Read the model definition and answer for the solid it produces. Units are mm, in the model's axes. Give positions to 0.01 mm unless a question says otherwise; leave off trailing zeros. Loops run counter-clockwise (first coordinate to the right, second up) from the corner with the lowest first, then second, coordinate; pieces in that order, holes last. Notation, with made-up numbers: (-9, 34) -> (48, 34) arc R38 ccw to (48, 73) -> close; hole circle Ø11 at (15.5, 24). An arc over 180 degrees is marked (long way). Return JSON: item names as keys, results as strings. Group by question number.
from build123d import *

# Parameters (mm, degrees)
SKETCH1_W           = 185
SKETCH1_H           = 100
SKETCH1_W_2         = 122
SKETCH1_H_2         = 30
BOSS_EXTRUDE1_DEPTH = 5
CUT_EXTRUDE2_REACH  = 7
SKETCH2_R           = 1.6
CUT_EXTRUDE3_REACH  = 7
SKETCH3_R           = 1.6
CUT_EXTRUDE4_REACH  = 7
SKETCH4_R           = 1.6
CUT_EXTRUDE5_REACH  = 7
SKETCH5_R           = 1.6


with BuildPart() as part:
    # Sketch1 → Boss-Extrude1 (new body)
    with BuildSketch(Plane(origin=(0, 0, 0), x_dir=(1, 0, 0), z_dir=(0, 1, 0))):
        with Locations((12.5, 9)):
            Rectangle(SKETCH1_W, SKETCH1_H)
        Rectangle(SKETCH1_W_2, SKETCH1_H_2, mode=Mode.SUBTRACT)
    extrude(amount=BOSS_EXTRUDE1_DEPTH)

    # Sketch2 → Cut-Extrude2 (cut, up to next)
    with BuildSketch(Plane(origin=(0, 0, 0), x_dir=(1, 0, 0), z_dir=(0, 1, 0)), mode=Mode.PRIVATE) as cut_extrude2_sk1:
        with Locations((-25, 20)):
            Circle(SKETCH2_R)
    cut_extrude2_tool1 = extrude(cut_extrude2_sk1.sketch, amount=CUT_EXTRUDE2_REACH, mode=Mode.PRIVATE) & part.part
    add(cut_extrude2_tool1.solids().sort_by_distance((-25, 0, -20))[0], mode=Mode.SUBTRACT)
    # Sketch2 → Cut-Extrude2 (cut, up to next)
    with BuildSketch(Plane(origin=(0, 0, 0), x_dir=(1, 0, 0), z_dir=(0, 1, 0)), mode=Mode.PRIVATE) as cut_extrude2_sk2:
        with Locations((25, 20)):
            Circle(SKETCH2_R)
    cut_extrude2_tool2 = extrude(cut_extrude2_sk2.sketch, amount=CUT_EXTRUDE2_REACH, mode=Mode.PRIVATE) & part.part
    add(cut_extrude2_tool2.solids().sort_by_distance((25, 0, -20))[0], mode=Mode.SUBTRACT)
    # Sketch2 → Cut-Extrude2 (cut, up to next)
    with BuildSketch(Plane(origin=(0, 0, 0), x_dir=(1, 0, 0), z_dir=(0, 1, 0)), mode=Mode.PRIVATE) as cut_extrude2_sk3:
        with Locations((25, -20)):
            Circle(SKETCH2_R)
    cut_extrude2_tool3 = extrude(cut_extrude2_sk3.sketch, amount=CUT_EXTRUDE2_REACH, mode=Mode.PRIVATE) & part.part
    add(cut_extrude2_tool3.solids().sort_by_distance((25, 0, 20))[0], mode=Mode.SUBTRACT)
    # Sketch2 → Cut-Extrude2 (cut, up to next)
    with BuildSketch(Plane(origin=(0, 0, 0), x_dir=(1, 0, 0), z_dir=(0, 1, 0)), mode=Mode.PRIVATE) as cut_extrude2_sk4:
        with Locations((-25, -20)):
            Circle(SKETCH2_R)
    cut_extrude2_tool4 = extrude(cut_extrude2_sk4.sketch, amount=CUT_EXTRUDE2_REACH, mode=Mode.PRIVATE) & part.part
    add(cut_extrude2_tool4.solids().sort_by_distance((-25, 0, 20))[0], mode=Mode.SUBTRACT)
    # Sketch2 → Cut-Extrude2 (cut, up to next)
    with BuildSketch(Plane(origin=(0, 0, 0), x_dir=(1, 0, 0), z_dir=(0, 1, 0)), mode=Mode.PRIVATE) as cut_extrude2_sk5:
        with Locations((-65, 20)):
            Circle(SKETCH2_R)
    cut_extrude2_tool5 = extrude(cut_extrude2_sk5.sketch, amount=CUT_EXTRUDE2_REACH, mode=Mode.PRIVATE) & part.part
    add(cut_extrude2_tool5.solids().sort_by_distance((-65, 0, -20))[0], mode=Mode.SUBTRACT)
    # Sketch2 → Cut-Extrude2 (cut, up to next)
    with BuildSketch(Plane(origin=(0, 0, 0), x_dir=(1, 0, 0), z_dir=(0, 1, 0)), mode=Mode.PRIVATE) as cut_extrude2_sk6:
        with Locations((65, 20)):
            Circle(SKETCH2_R)
    cut_extrude2_tool6 = extrude(cut_extrude2_sk6.sketch, amount=CUT_EXTRUDE2_REACH, mode=Mode.PRIVATE) & part.part
    add(cut_extrude2_tool6.solids().sort_by_distance((65, 0, -20))[0], mode=Mode.SUBTRACT)
    # Sketch2 → Cut-Extrude2 (cut, up to next)
    with BuildSketch(Plane(origin=(0, 0, 0), x_dir=(1, 0, 0), z_dir=(0, 1, 0)), mode=Mode.PRIVATE) as cut_extrude2_sk7:
        with Locations((65, -20)):
            Circle(SKETCH2_R)
    cut_extrude2_tool7 = extrude(cut_extrude2_sk7.sketch, amount=CUT_EXTRUDE2_REACH, mode=Mode.PRIVATE) & part.part
    add(cut_extrude2_tool7.solids().sort_by_distance((65, 0, 20))[0], mode=Mode.SUBTRACT)
    # Sketch2 → Cut-Extrude2 (cut, up to next)
    with BuildSketch(Plane(origin=(0, 0, 0), x_dir=(1, 0, 0), z_dir=(0, 1, 0)), mode=Mode.PRIVATE) as cut_extrude2_sk8:
        with Locations((-65, -20)):
            Circle(SKETCH2_R)
    cut_extrude2_tool8 = extrude(cut_extrude2_sk8.sketch, amount=CUT_EXTRUDE2_REACH, mode=Mode.PRIVATE) & part.part
    add(cut_extrude2_tool8.solids().sort_by_distance((-65, 0, 20))[0], mode=Mode.SUBTRACT)

    # Sketch3 → Cut-Extrude3 (cut, up to next)
    with BuildSketch(Plane(origin=(0, 5, 0), x_dir=(1, 0, 0), z_dir=(0, 1, 0)), mode=Mode.PRIVATE) as cut_extrude3_sk1:
        with Locations((-27.5, 39)):
            Circle(SKETCH3_R)
    cut_extrude3_tool1 = extrude(cut_extrude3_sk1.sketch, amount=-CUT_EXTRUDE3_REACH, mode=Mode.PRIVATE) & part.part
    add(cut_extrude3_tool1.solids().sort_by_distance((-27.5, 5, -39))[0], mode=Mode.SUBTRACT)
    # Sketch3 → Cut-Extrude3 (cut, up to next)
    with BuildSketch(Plane(origin=(0, 5, 0), x_dir=(1, 0, 0), z_dir=(0, 1, 0)), mode=Mode.PRIVATE) as cut_extrude3_sk2:
        with Locations((-12.5, 39)):
            Circle(SKETCH3_R)
    cut_extrude3_tool2 = extrude(cut_extrude3_sk2.sketch, amount=-CUT_EXTRUDE3_REACH, mode=Mode.PRIVATE) & part.part
    add(cut_extrude3_tool2.solids().sort_by_distance((-12.5, 5, -39))[0], mode=Mode.SUBTRACT)
    # Sketch3 → Cut-Extrude3 (cut, up to next)
    with BuildSketch(Plane(origin=(0, 5, 0), x_dir=(1, 0, 0), z_dir=(0, 1, 0)), mode=Mode.PRIVATE) as cut_extrude3_sk3:
        with Locations((37.5, 39)):
            Circle(SKETCH3_R)
    cut_extrude3_tool3 = extrude(cut_extrude3_sk3.sketch, amount=-CUT_EXTRUDE3_REACH, mode=Mode.PRIVATE) & part.part
    add(cut_extrude3_tool3.solids().sort_by_distance((37.5, 5, -39))[0], mode=Mode.SUBTRACT)
    # Sketch3 → Cut-Extrude3 (cut, up to next)
    with BuildSketch(Plane(origin=(0, 5, 0), x_dir=(1, 0, 0), z_dir=(0, 1, 0)), mode=Mode.PRIVATE) as cut_extrude3_sk4:
        with Locations((52.5, 39)):
            Circle(SKETCH3_R)
    cut_extrude3_tool4 = extrude(cut_extrude3_sk4.sketch, amount=-CUT_EXTRUDE3_REACH, mode=Mode.PRIVATE) & part.part
    add(cut_extrude3_tool4.solids().sort_by_distance((52.5, 5, -39))[0], mode=Mode.SUBTRACT)

    # Sketch4 → Cut-Extrude4 (cut, up to next)
    with BuildSketch(Plane(origin=(0, 5, 0), x_dir=(1, 0, 0), z_dir=(0, 1, 0)), mode=Mode.PRIVATE) as cut_extrude4_sk1:
        with Locations((-37.5, -28.5)):
            Circle(SKETCH4_R)
    cut_extrude4_tool1 = extrude(cut_extrude4_sk1.sketch, amount=-CUT_EXTRUDE4_REACH, mode=Mode.PRIVATE) & part.part
    add(cut_extrude4_tool1.solids().sort_by_distance((-37.5, 5, 28.5))[0], mode=Mode.SUBTRACT)
    # Sketch4 → Cut-Extrude4 (cut, up to next)
    with BuildSketch(Plane(origin=(0, 5, 0), x_dir=(1, 0, 0), z_dir=(0, 1, 0)), mode=Mode.PRIVATE) as cut_extrude4_sk2:
        with Locations((37.5, -28.5)):
            Circle(SKETCH4_R)
    cut_extrude4_tool2 = extrude(cut_extrude4_sk2.sketch, amount=-CUT_EXTRUDE4_REACH, mode=Mode.PRIVATE) & part.part
    add(cut_extrude4_tool2.solids().sort_by_distance((37.5, 5, 28.5))[0], mode=Mode.SUBTRACT)

    # Sketch5 → Cut-Extrude5 (cut, up to next)
    with BuildSketch(Plane.XZ, mode=Mode.PRIVATE) as cut_extrude5_sk1:
        with Locations((85, -1.5)):
            Circle(SKETCH5_R)
    cut_extrude5_tool1 = extrude(cut_extrude5_sk1.sketch, amount=-CUT_EXTRUDE5_REACH, mode=Mode.PRIVATE) & part.part
    add(cut_extrude5_tool1.solids().sort_by_distance((85, 0, -1.5))[0], mode=Mode.SUBTRACT)
    # Sketch5 → Cut-Extrude5 (cut, up to next)
    with BuildSketch(Plane.XZ, mode=Mode.PRIVATE) as cut_extrude5_sk2:
        with Locations((85, -16.5)):
            Circle(SKETCH5_R)
    cut_extrude5_tool2 = extrude(cut_extrude5_sk2.sketch, amount=-CUT_EXTRUDE5_REACH, mode=Mode.PRIVATE) & part.part
    add(cut_extrude5_tool2.solids().sort_by_distance((85, 0, -16.5))[0], mode=Mode.SUBTRACT)


solid = part.part
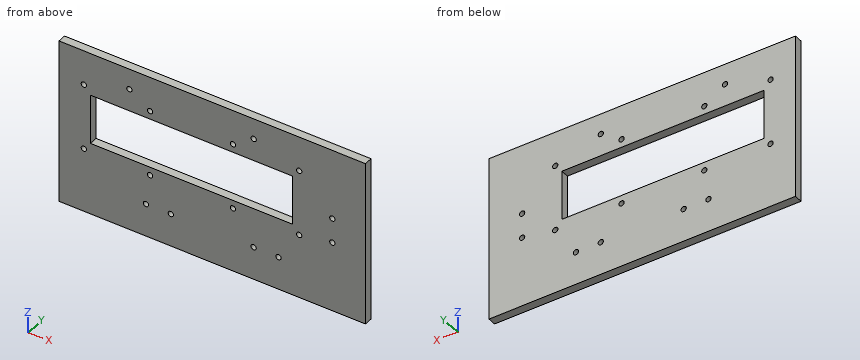
1. A flat-ended cylindrical pin translates along its axis: pin 1 Ø1.9 at (x, z) = (65, -20) entering from +Y. Find the tip coordinate at first contact, or state that the pin passes through.
2. Section A-A on x = 56.5 is taken. Determine the outline of the cut face in (y, z).
3. Straight lines are drawn through the part: line 1 (X direction, y = 2.4, z = -20); line 2 (Z direction, x = 52.5, y = 1.05); line 3 (Z direction, x = -25, y = 3.95). For each, find the intervals that lie inside material, in ascending order. Write a range as from..to.
Completed:
{
 "1": {"pin 1": "passes through"},
 "2": {"outline": "(0, -59) -> (5, -59) -> (5, -15) -> (0, -15) -> close; (0, 15) -> (5, 15) -> (5, 41) -> (0, 41) -> close"},
 "3": {"line 1": "x = -80..-66.6, -63.4..-26.6, -23.4..23.4, 26.6..63.4, 66.6..105", "line 2": "z = -59..-40.6, -37.4..-15, 15..41", "line 3": "z = -59..-21.6, -18.4..-15, 15..18.4, 21.6..41"}
}
